Here's how the part is built. I have some questions about the finished solid (model axes, mm). A direction names the side the tool comes from. Round coordinates to 2 decimals unless told otherwise and drop trailing zeros. Loops run counter-clockwise (first coordinate to the right, second up) from the corner with the lowest first, then second, coordinate; pieces in that order, holes last. Notation, with made-up numbers: (52.25, 83.5) -> (93.25, 83.5) arc R17 cw to (93.25, 114.5) -> close; hole circle Ø6 at (64, 38.25). An arc over 180 degrees is marked (long way). One line per item, written item: value. Start each with the question number.
```python
from build123d import *

# Parameters (mm, degrees)
SKETCH1_W           = 90
SKETCH1_H           = 30
BOSS_EXTRUDE1_DEPTH = 3
SKETCH2_R           = 1.5
CUT_EXTRUDE1_DEPTH  = 3
SKETCH3_W           = 3
SKETCH3_H           = 30
BOSS_EXTRUDE2_DEPTH = 7
SKETCH4_R           = 1.5
CUT_EXTRUDE2_DEPTH  = 7
SKETCH5_W           = 67
SKETCH5_H           = 5
CUT_EXTRUDE3_DEPTH  = 7
FILLET1_START       = -7
FILLET1_DEPTH       = 11
FILLET1_2_DEPTH     = 3
SKETCH6_R           = 3
CUT_EXTRUDE4_DEPTH  = 10


with BuildPart() as part:
    # Sketch1 → Boss-Extrude1 (new body)
    with BuildSketch(Plane.XY):
        Rectangle(SKETCH1_W, SKETCH1_H)
    extrude(amount=BOSS_EXTRUDE1_DEPTH)

    # Sketch2 → Cut-Extrude1 (cut)
    with BuildSketch(Plane.XY.offset(3)):
        with Locations((-38, 10)):
            Circle(SKETCH2_R)
    cut_extrude1 = extrude(amount=-CUT_EXTRUDE1_DEPTH, mode=Mode.SUBTRACT)

    # Sketch3 → Boss-Extrude2 (add)
    with BuildSketch(Plane(origin=(0, 0, 0), x_dir=(-1, 0, 0), z_dir=(0, 0, -1))):
        with Locations((-43.5, 0)):
            Rectangle(SKETCH3_W, SKETCH3_H)
    extrude(amount=BOSS_EXTRUDE2_DEPTH)

    # Sketch4 → Cut-Extrude2 (cut)
    with BuildSketch(Plane.ZY.offset(-42)):
        with Locations((-4, 10)):
            Circle(SKETCH4_R)
    cut_extrude2 = extrude(amount=-CUT_EXTRUDE2_DEPTH, mode=Mode.SUBTRACT)

    # Sketch5 → Cut-Extrude3 (cut)
    with BuildSketch(Plane.XY.offset(3)):
        with Locations((1.5, 12.5)):
            Rectangle(SKETCH5_W, SKETCH5_H)
    cut_extrude3 = extrude(amount=-CUT_EXTRUDE3_DEPTH, mode=Mode.SUBTRACT)

    # Mirror1: Cut-Extrude1, Cut-Extrude2, Cut-Extrude3 across plane
    add(cut_extrude1.mirror(Plane.ZX), mode=Mode.SUBTRACT)
    add(cut_extrude2.mirror(Plane.ZX), mode=Mode.SUBTRACT)
    add(cut_extrude3.mirror(Plane.ZX), mode=Mode.SUBTRACT)

    # Fillet1: read off the stored shape, not the designer's step
    # Fillet1 outline → Fillet1 (cut)
    with BuildSketch(Plane.XY.offset(FILLET1_START)):
        with BuildLine():
            Line((-32, -15), (-32, -12.5))
            ThreePointArc((-32, -12.5), (-32.732233047, -14.267766953), (-34.5, -15))
            Line((-34.5, -15), (-32, -15))
        make_face()
        with BuildLine():
            ThreePointArc((37.5, -15), (35.732233047, -14.267766953), (35, -12.5))
            Line((35, -12.5), (35, -15))
            Line((35, -15), (37.5, -15))
        make_face()
        with BuildLine():
            ThreePointArc((-34.5, 15), (-32.732233047, 14.267766953), (-32, 12.5))
            Line((-32, 12.5), (-32, 15))
            Line((-32, 15), (-34.5, 15))
        make_face()
        with BuildLine():
            ThreePointArc((35, 12.5), (35.732233047, 14.267766953), (37.5, 15))
            Line((37.5, 15), (35, 15))
            Line((35, 15), (35, 12.5))
        make_face()
    extrude(amount=FILLET1_DEPTH, mode=Mode.SUBTRACT)

    # Fillet1 2 outline → Fillet1 2 (add)
    with BuildSketch(Plane.XY):
        with BuildLine():
            Line((35, -10), (32.5, -10))
            ThreePointArc((32.5, -10), (34.267766953, -10.732233047), (35, -12.5))
            Line((35, -12.5), (35, -10))
        make_face()
        with BuildLine():
            ThreePointArc((-32, -12.5), (-31.267766953, -10.732233047), (-29.5, -10))
            Line((-29.5, -10), (-32, -10))
            Line((-32, -10), (-32, -12.5))
        make_face()
        with BuildLine():
            Line((-32, 10), (-29.5, 10))
            ThreePointArc((-29.5, 10), (-31.267766953, 10.732233047), (-32, 12.5))
            Line((-32, 12.5), (-32, 10))
        make_face()
        with BuildLine():
            Line((35, 10), (35, 12.5))
            ThreePointArc((35, 12.5), (34.267766953, 10.732233047), (32.5, 10))
            Line((32.5, 10), (35, 10))
        make_face()
    extrude(amount=FILLET1_2_DEPTH)

    # Sketch6 → Cut-Extrude4 (cut)
    with BuildSketch(Plane.XY.offset(3)):
        with Locations((25, 0)):
            Circle(SKETCH6_R)
    extrude(amount=-CUT_EXTRUDE4_DEPTH, mode=Mode.SUBTRACT)


solid = part.part
```
Q1. I want a section at A-A on x = 25. Please give me the cut outline in (y, z), plus the area to 3 significant figures.
Q2. I want a section at C-C on z = -4. Please give me the cut outline in (x, y), plus the area to 3 significant figures.
Q3. If I drill on line 1 along Y through (x, z) = (44.25, -4); line 2 along X through (y, z) = (-0.25, 2.75); line 3 along Z through (x, y) = (-3.5, -3.5), over which ranges is the centre line in solid material (lowest first)?
Q4. I want a section at B-B on y = 0. Please give me the cut outline in (x, z), plus the area to 3 significant figures.
Q5. I want a section at D-D on x = -38. Please give me the cut outline in (y, z), plus the area to 3 significant figures.
Q6. Will these pins go through, and if not, where does the flat tip stop? P1, Ø0.9, axis at x = 6, z = 1, coming from the +Y side; P2, Ø2, axis at y = -11, z = -4.5, coming from the +X side; P3, Ø2.5, axis at x = -5, z = 1.5, coming from the -Y side; P4, Ø5, axis at x = 28, y = 10, coming from the -Z side.
Q7. If we mould it in two halves opening along Z, with no side actions, what happens to faces 4 (the flat face through (-2, 0, 0)), 5 (the flat face through (-40, 15, 2)), 6 (the cylindrical face through (43.479, 9.425, -2.614))? For each: released by +Z, released by -Z, zero draft, split by the parting line, or undercut.
Q8. Which directions (+Z, -Z, +X, -X, +Y, -Y) give clear straight access to the entire face, cutting with the end or side of a thin tool? Please do faces 1 (the flat face through (1, 10, 2)), 2 (the flat face through (42, 0, -3)), 3 (the flat face through (1, -10, 2)).
Answers below:
1. outline: (-10, 0) -> (-3, 0) -> (-3, 3) -> (-10, 3) -> close; (3, 0) -> (10, 0) -> (10, 3) -> (3, 3) -> close
1. area: 42.0 mm^2
2. outline: (42, -15) -> (45, -15) -> (45, -11.5) -> (42, -11.5) -> close; (42, -8.5) -> (45, -8.5) -> (45, 8.5) -> (42, 8.5) -> close; (42, 11.5) -> (45, 11.5) -> (45, 15) -> (42, 15) -> close
2. area: 72.0 mm^2
3. line 1: y = -15 to -11.5, -8.5 to 8.5, 11.5 to 15
3. line 2: x = -45 to 22.01, 27.99 to 45
3. line 3: z = 0 to 3
4. outline: (-45, 0) -> (22, 0) -> (22, 3) -> (-45, 3) -> close; (28, 0) -> (42, 0) -> (42, -7) -> (45, -7) -> (45, 3) -> (28, 3) -> close
4. area: 273 mm^2
5. outline: (-15, 0) -> (-11.5, 0) -> (-11.5, 3) -> (-15, 3) -> close; (-8.5, 0) -> (8.5, 0) -> (8.5, 3) -> (-8.5, 3) -> close; (11.5, 0) -> (15, 0) -> (15, 3) -> (11.5, 3) -> close
5. area: 72.0 mm^2
6. P1: stops at y = 10
6. P2: stops at x = 45
6. P3: stops at y = -10
6. P4: stops at z = 0
7. face 4: released by -Z
7. face 5: zero draft
7. face 6: undercut
8. face 1: +Z, -Z, +Y
8. face 2: -Z, -X, +Y, -Y
8. face 3: +Z, -Z, -Y
